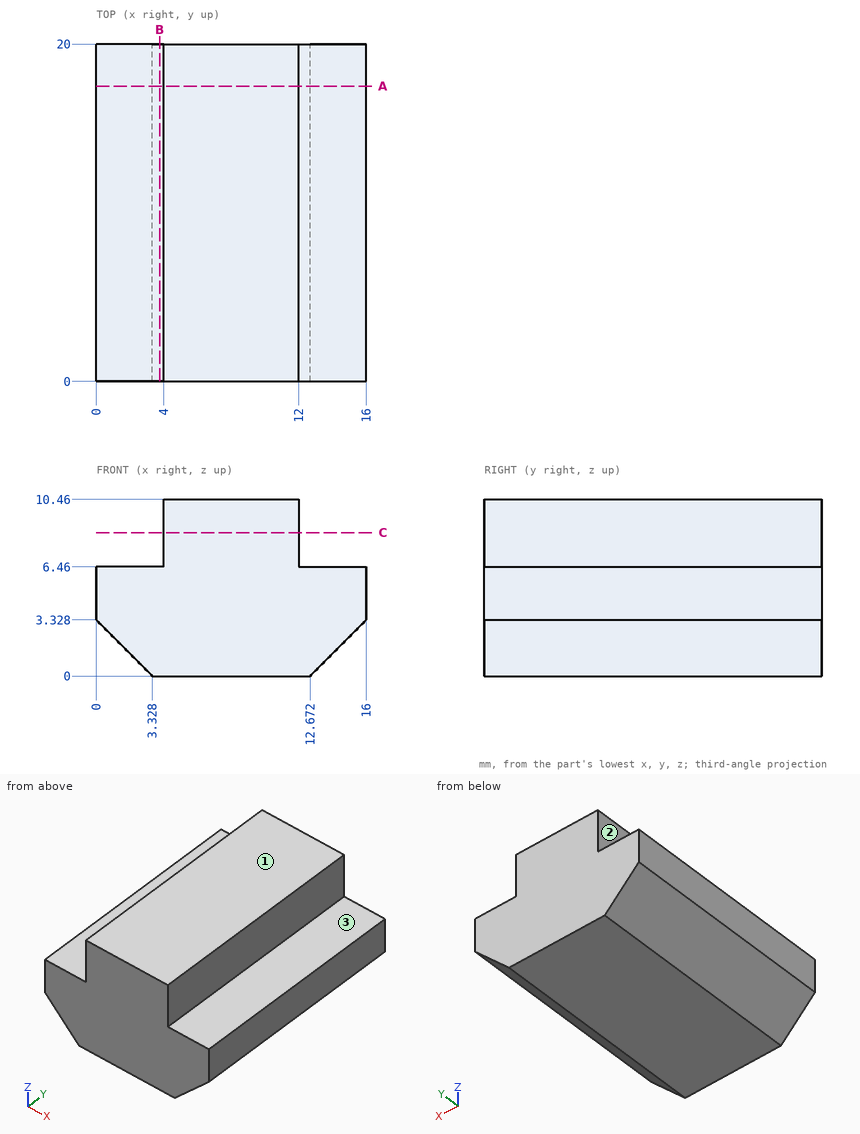
Geometry check sheet. Reference: drawing and pictorial views, mm from the part's lowest x, y, z. A direction names the side the tool comes from. Round coordinates to 2 decimals unless told otherwise and drop trailing zeros. Order: outer loops, then holes, each group sorted by start corner. A loop starts at its lowest first (then second) coordinate and runs counter-clockwise, first axis right, second up. Notation, with made-up numbers: (-0.75, 80.25) - (37.25, 80.25) arc R8 ccw to (37.25, 92.25) - close; hole circle Ø1 at (11, 63.25). An arc over 180 degrees is marked (long way). Use a Markdown table: item, result. Add a question column.
1) Thickness scan on line 1 along X through (y, z) = (2, 9.25); line 2 along Z through (x, y) = (3.75, 8.75); line 3 along X through (y, z) = (11.25, 0.5). Record the ranges inside material, lowest first.
2) Gauge pin test, flat ends, axial feed: P1, Ø3, axis at x = 1.5, y = 9, coming from the +Z side; P2, Ø3, axis at y = 15, z = 8.5, coming from the -X side; P3, Ø1.5, axis at y = 10.5, z = 2.5, coming from the -X side. Record the tip position at first contact, or that the pin passes through.
3) Section check B-B (x = 3.75). Record the cut outline in (y, z), then the cut area to 3 significant figures.
4) Section check C-C (z = 8.5). Record the cut outline in (x, y).
5) Section check A-A (y = 17.5). Record the cut outline in (x, z), then the cut area to 3 significant figures.
6) Set-up check for the marked faces 1, 2 and 3: record each of +Z, -Z, +X, -X, +Y, -Y from which the full face is reachable in a straight line by a thin tool's end or side.
Established:
| question | item | result |
|---|---|---|
| 1 | line 1 | 4 to 12 |
| 1 | line 2 | 0 to 6.46 |
| 1 | line 3 | 2.83 to 13.17 |
| 2 | P1 | z = 6.46 |
| 2 | P2 | x = 4 |
| 2 | P3 | x = 0.08 |
| 3 | outline | (0, 0) - (20, 0) - (20, 6.46) - (0, 6.46) - close |
| 3 | area | 129 mm2 |
| 4 | outline | (4, 0) - (12, 0) - (12, 20) - (4, 20) - close |
| 5 | outline | (0, 3.33) - (3.33, 0) - (12.67, 0) - (16, 3.33) - (16, 6.46) - (12, 6.46) - (12, 10.46) - (4, 10.46) - (4, 6.46) - (0, 6.46) - close |
| 5 | area | 124 mm2 |
| 6 | face 1 | +Z, +X, -X, +Y, -Y |
| 6 | face 2 | +Z, -X, +Y, -Y |
| 6 | face 3 | +Z, +X, +Y, -Y |
